CAD build for the part. Positions are in the model's coordinates, mm. A direction names the side the tool comes from. Give positions to 0.01 mm unless a question says otherwise; leave off trailing zeros. Write each loop counter-clockwise with the first axis right and the second up, starting at its lowest first coordinate (ties: lowest second). Pieces come first, ordered by that corner, then holes. Notation, with made-up numbers: (71, 4) - (75, 4) arc R17 cw to (75, 14) - close; hole circle Ø1 at (-20.75, 13). An arc over 180 degrees is marked (long way). Put each result on its own line as item: value. Start each with the question number.
1. Cut at C-C on x = 46. List the corners of the cut face in (y, z).
2. Tool access for faces 1 (the flat face through (28, 42, 19)), 2 (the cylindrical face through (14.24, 18.983, 38.507)), 3 (the flat face through (53, 11, 54)): list every direction of +Z, -Z, +X, -X, +Y, -Y with a clear straight run to the whole face (end or side of a thin tool).
3. Cut at B-B on z = 44.5. List the corners of the cut face in (x, y).
4. Drop flat-ended pins along their axis: pin 1 (2.5 mm diameter, centred on x = 40.5, y = 17, fed in from -Z); pin 2 (4 mm diameter, centred on x = 8.5, y = 17, fed in from +Z); pin 3 (4 mm diameter, centred on x = 29, z = 46.5, fed in from +Y). Give the stop position or say it passes through.
5. Cut at A-A on y = 28. List the corners of the cut face in (x, z).
6. Cut at D-D on z = 7.5. List the corners of the cut face in (x, y).
7. Wall check: line 1 (X direction, y = 3.3, z = 75.5); line 2 (X direction, y = 14.5, z = 49.5); line 3 (Z direction, x = 8.5, y = 1.45). Give the ranges that are in metal, low to high.
8. Mould opens along X. For faces 4 (the flat face through (54, 21, 44)), 5 (the cylindrical face through (16, 17, 19)), 6 (the flat face through (0, 12, 32)) say: +X half, -X half, draft (parallel to the pull), parting line (faces both ways), or undercut.
from build123d import *

# Parameters (mm, degrees)
BOSS_EXTRUDE1_DEPTH = 39
SKETCH2_W           = 55
SKETCH2_H           = 5
BOSS_EXTRUDE2_DEPTH = 42
SKETCH3_R           = 11.5
SKETCH3_R_2         = 1.5
SKETCH3_R_3         = 4
CUT_EXTRUDE1_DEPTH  = 105.66613588
SKETCH4_R           = 1.5
CUT_EXTRUDE2_DEPTH  = 81.950602221
SKETCH5_R           = 2
CUT_EXTRUDE3_DEPTH  = 1
SKETCH6_W           = 2
SKETCH6_H           = 42
BOSS_EXTRUDE3_DEPTH = 16
CUT_EXTRUDE4_DEPTH  = 100


with BuildPart() as part:
    # Sketch1 → Boss-Extrude1 (new body)
    with BuildSketch(Plane.XY):
        Polygon((0, 0), (55, 0), (55, 32), (37.5, 42), (17.5, 42), (0, 32), align=None)
    extrude(amount=BOSS_EXTRUDE1_DEPTH)

    # Sketch2 → Boss-Extrude2 (add)
    with BuildSketch(Plane.XY.offset(39)):
        with Locations((27.5, 2.5)):
            Rectangle(SKETCH2_W, SKETCH2_H)
    extrude(amount=BOSS_EXTRUDE2_DEPTH)

    # Sketch3 → Cut-Extrude1 (cut, through all)
    with BuildSketch(Plane(origin=(0, 5, 0), x_dir=(1, 0, 0), z_dir=(0, 1, 0))):
        with Locations(Location((24, -60, 0), (0, 0, 180))):
            Circle(SKETCH3_R)
        with Locations(Location((8.5, -44.5, 0), (0, 0, 180))):
            Circle(SKETCH3_R_2)
        with Locations(Location((39.5, -44.5, 0), (0, 0, 180))):
            Circle(SKETCH3_R_2)
        with Locations(Location((39.5, -75.5, 0), (0, 0, 180))):
            Circle(SKETCH3_R_2)
        with Locations(Location((8.5, -75.5, 0), (0, 0, 180))):
            Circle(SKETCH3_R_2)
        with Locations(Location((46, -60, 0), (0, 0, 180))):
            Circle(SKETCH3_R_3)
    extrude(amount=-CUT_EXTRUDE1_DEPTH, mode=Mode.SUBTRACT)

    # Sketch4 → Cut-Extrude2 (cut, through all)
    with BuildSketch(Plane.XY.offset(39)):
        with Locations((27.5, 28)):
            Circle(SKETCH4_R)
        with Locations((40.5, 17)):
            Circle(SKETCH4_R)
        with Locations(Location((14.5, 17, 0), (0, 0, 180))):
            Circle(SKETCH4_R)
    extrude(amount=-CUT_EXTRUDE2_DEPTH, mode=Mode.SUBTRACT)

    # Sketch5 → Cut-Extrude3 (cut)
    with BuildSketch(Plane.XY.offset(39)):
        with Locations((27.5, 28)):
            Circle(SKETCH5_R)
        with Locations((40.5, 17)):
            Circle(SKETCH5_R)
        with Locations((14.5, 17)):
            Circle(SKETCH5_R)
    extrude(amount=-CUT_EXTRUDE3_DEPTH, mode=Mode.SUBTRACT)

    # Sketch6 → Boss-Extrude3 (add)
    with BuildSketch(Plane(origin=(0, 5, 0), x_dir=(1, 0, 0), z_dir=(0, 1, 0))):
        with Locations((1, -60)):
            Rectangle(SKETCH6_W, SKETCH6_H)
        with Locations((54, -60)):
            Rectangle(SKETCH6_W, SKETCH6_H)
    extrude(amount=BOSS_EXTRUDE3_DEPTH)

    # Sketch7 → Cut-Extrude4 (cut)
    with BuildSketch(Plane(origin=(55, 0, 0), x_dir=(0, 0, -1), z_dir=(1, 0, 0))):
        Polygon((-49, 21), (-81, 21), (-81, 2), align=None)
    extrude(amount=-CUT_EXTRUDE4_DEPTH, mode=Mode.SUBTRACT)


solid = part.part
Report:
1. outline: (0, 0) - (37.14, 0) - (37.14, 39) - (5, 39) - (5, 56) - (0, 56) - close; (0, 64) - (5, 64) - (5, 75.95) - (2, 81) - (0, 81) - close
2. face 1: +Z, -Z, +X, -X, +Y
2. face 2: +Z
2. face 3: +Z, +Y
3. outline: (0, 0) - (7, 0) - (7, 5) - (2, 5) - (2, 21) - (0, 21) - close; (10, 0) - (38, 0) - (38, 5) - (10, 5) - close; (41, 0) - (55, 0) - (55, 21) - (53, 21) - (53, 5) - (41, 5) - close
4. pin 1: passes through
4. pin 2: stops at z = 39
4. pin 3: stops at y = 5
5. outline: (0, 0) - (26, 0) - (26, 38) - (25.5, 38) - (25.5, 39) - (0, 39) - close; (29, 0) - (55, 0) - (55, 39) - (29.5, 39) - (29.5, 38) - (29, 38) - close
6. outline: (0, 0) - (55, 0) - (55, 32) - (37.5, 42) - (17.5, 42) - (0, 32) - close; hole circle Ø3 at (14.5, 17); hole circle Ø3 at (27.5, 28); hole circle Ø3 at (40.5, 17)
7. line 1: x = 0 to 7, 10 to 38, 41 to 55
7. line 2: x = 0 to 2, 53 to 55
7. line 3: z = 0 to 43, 46 to 74, 77 to 81
8. face 4: draft
8. face 5: undercut
8. face 6: -X half
